The model under review builds one solid part; all positions refer to its coordinate system, in mm. Face numbers are marked on the shaded views. Coordinates: 2 decimals unless noted, no trailing zeros. Write each loop counter-clockwise with the first axis right and the second up, starting at its lowest first coordinate (ties: lowest second). Pieces come first, ordered by that corner, then holes. Notation, with made-up numbers: (43, 63.5) - (56, 63.5) arc R29 cw to (56, 90.5) - close; hole circle Ø4 at (89, 28.25). An arc over 180 degrees is marked (long way). Return JSON: item names as keys, results as strings. Group by question number.
(1) To check wall thickness, follow L1, parallel to Y at x = 0, z = 2.6; L2, parallel to Y at x = -7, z = 1.5; L3, parallel to X at y = -4.5, z = 0.9. State the ranges of each line that lie inside material, in increasing order. Write a range as from..to.
(2) We need section D-D on y = -9. State the section outline as (x, z) points.
(3) Draft analysis for pull direction X (two halves, no side actions). For the marked faces 1, 2 and 3, state which applies: released by +X, released by -X, zero draft, split by the parting line, or undercut.
(4) We need section C-C on x = 0. State the section outline as (y, z) points.
(5) We need section A-A on z = 3.4. State the section outline as (x, y) points, then the cut area to 3 significant figures.
(6) We need section B-B on y = 6. State the section outline as (x, z) points.
(7) For pin 1 Ø1.5 at (x, z) = (-0.5, 2) entering from -Y; pin 2 Ø3 at (y, z) = (11, 1) entering from -X; pin 3 Ø3 at (x, z) = (-3, 1) entering from +Y, all flat-tipped, find the tip position at first contact; note any pin that passes through.
```python
from build123d import *

# Parameters (mm, degrees)
SKETCH_1_R          = 21
EXTRUDE_1_DEPTH     = 2
SKETCH_2_R          = 20
EXTRUDE_2_DEPTH     = 3
SKETCH_3_R          = 2
CUT_EXTRUDE_1_DEPTH = 31.116440693


with BuildPart() as part:
    # 草图1 → 凸台-拉伸1 (new body)
    with BuildSketch(Plane.XY):
        Circle(SKETCH_1_R)
    extrude(amount=EXTRUDE_1_DEPTH)

    # 草图2 → 凸台-拉伸2 (add)
    with BuildSketch(Plane.XY.offset(2)):
        Circle(SKETCH_2_R)
    extrude(amount=EXTRUDE_2_DEPTH)

    # 草图3 → 切除-拉伸1 (cut, through all)
    with BuildSketch(Plane.XY.offset(5)):
        with Locations((0, 10)):
            Circle(SKETCH_3_R)
        with Locations((8.660254038, 5)):
            Circle(SKETCH_3_R)
        with Locations((8.660254038, -5)):
            Circle(SKETCH_3_R)
        with Locations((0, -10)):
            Circle(SKETCH_3_R)
        with Locations((-8.660254038, -5)):
            Circle(SKETCH_3_R)
        with Locations((-8.660254038, 5)):
            Circle(SKETCH_3_R)
    extrude(amount=-CUT_EXTRUDE_1_DEPTH, mode=Mode.SUBTRACT)


solid = part.part
```
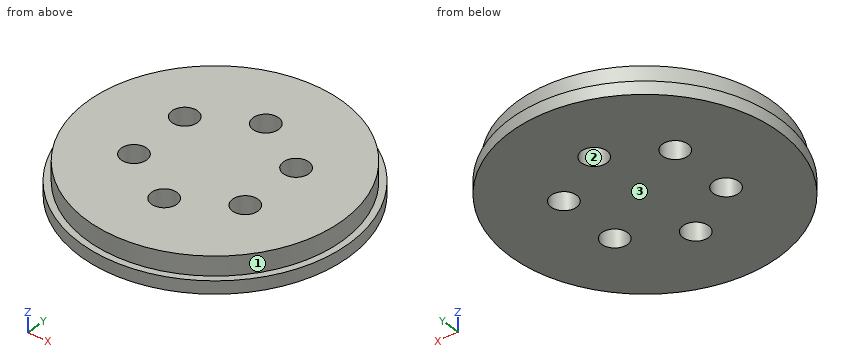
Ans:
{
 "1": {"L1": "-20..-12, -8..8, 12..20", "L2": "-19.8..-6.12, -3.88..3.88, 6.12..19.8", "L3": "-20.51..-10.6, -6.72..6.72, 10.6..20.51"},
 "2": {"outline": "(-18.97, 0) - (-1.73, 0) - (-1.73, 5) - (-17.86, 5) - (-17.86, 2) - (-18.97, 2) - close; (1.73, 0) - (18.97, 0) - (18.97, 2) - (17.86, 2) - (17.86, 5) - (1.73, 5) - close"},
 "3": {"face 1": "split by the parting line", "face 2": "undercut", "face 3": "zero draft"},
 "4": {"outline": "(-21, 0) - (-12, 0) - (-12, 5) - (-20, 5) - (-20, 2) - (-21, 2) - close; (-8, 0) - (8, 0) - (8, 5) - (-8, 5) - close; (12, 0) - (21, 0) - (21, 2) - (20, 2) - (20, 5) - (12, 5) - close"},
 "5": {"outline": "circle Ø40 at (0, 0); hole circle Ø4 at (-8.66, -5); hole circle Ø4 at (-8.66, 5); hole circle Ø4 at (0, -10); hole circle Ø4 at (0, 10); hole circle Ø4 at (8.66, -5); hole circle Ø4 at (8.66, 5)", "area": "1,180 mm²"},
 "6": {"outline": "(-20.12, 0) - (-10.39, 0) - (-10.39, 5) - (-19.08, 5) - (-19.08, 2) - (-20.12, 2) - close; (-6.93, 0) - (6.93, 0) - (6.93, 5) - (-6.93, 5) - close; (10.39, 0) - (20.12, 0) - (20.12, 2) - (19.08, 2) - (19.08, 5) - (10.39, 5) - close"},
 "7": {"pin 1": "y = -21", "pin 2": "x = -18.73", "pin 3": "y = 20.95"}
}
